from build123d import *

# Parameters (mm, degrees)
SKETCH1_R          = 2.54
EXTRUDE1_DEPTH     = 30.48
SKETCH2_W          = 2.032
SKETCH2_H          = 9.951877561
SKETCH2_W_2        = 1.949333431
SKETCH2_H_2        = 9.106721584
CUT_EXTRUDE1_DEPTH = 10.16
SKETCH4_R          = 1.524
CUT_EXTRUDE2_DEPTH = 10


with BuildPart() as part:
    # Sketch1 → Extrude1 (new body)
    with BuildSketch(Plane(origin=(0, 0, 0), x_dir=(1, 0, 0), z_dir=(0, 1, 0))):
        Circle(SKETCH1_R)
    extrude(amount=EXTRUDE1_DEPTH)

    # Sketch2 → Cut-Extrude1 (cut)
    with BuildSketch(Plane(origin=(0, 30.48, 0), x_dir=(-1, 0, 0), z_dir=(0, 1, 0))):
        with Locations((-2.54, 0.177802653)):
            Rectangle(SKETCH2_W, SKETCH2_H)
        with Locations((2.498666716, 0.600380641)):
            Rectangle(SKETCH2_W_2, SKETCH2_H_2)
    extrude(amount=-CUT_EXTRUDE1_DEPTH, mode=Mode.SUBTRACT)

    # Sketch4 → Cut-Extrude2 (cut)
    with BuildSketch(Plane.ZY.offset(1.524)):
        with Locations((0, 27.432)):
            Circle(SKETCH4_R)
    extrude(amount=-CUT_EXTRUDE2_DEPTH, mode=Mode.SUBTRACT)


solid = part.part
Work out the finished part from the listing and answer in its coordinate system (mm). A direction names the side the tool comes from. Round coordinates to 2 decimals unless told otherwise and drop trailing zeros. Write each loop counter-clockwise with the first axis right and the second up, starting at its lowest first coordinate (ties: lowest second). Pieces come first, ordered by that corner, then holes. Notation, with made-up numbers: (88, 75.25) -> (116, 75.25) arc R31 ccw to (116, 103.25) -> close; hole circle Ø1 at (-38, 2). An arc over 180 degrees is marked (long way). Answer as CSV lines item,"result". Start each with the question number.
(1) The part is cut by section B-B, the plane x = -0.05. Give the vertices of the cut face in (y, z), then the cut area to 3 significant figures.
(2) The part is cut by section A-A, the plane z = 0. Give the vertices of the cut face in (x, y).
(3) The part is cut by section C-C, the plane y = 25.5. Give the vertices of the cut face in (x, z).
(4) Find the intervals of material crossed by probe 1 along Y at (x, z) = (0.85, 0); probe 2 along Y at (x, z) = (-2.2, -1.15); probe 3 along Z at (x, y) = (-0.65, 26.5), in increasing order.
(5) The mould has two halves that part along Y. Classify faces 4 (the cylindrical face through (-0.021, 25.944, -0.33)), 5 (the flat face through (0, 30.48, 0)), 6 (the flat face through (-1.524, 25, 0)): +Y half, -Y half, draft (parallel to the pull), parting line (faces both ways), or undercut.
(6) Each of these flat-tipped pins is pushed along its axis until it touches: pin 1 (0.5 mm diameter, centred on x = -2, z = -0.5, fed in from +Y); pin 2 (1.5 mm diameter, centred on y = 9.5, z = -1.5, fed in from +X); pin 3 (1 mm diameter, centred on x = -2, y = 5.5, fed in from -Z). Where does it stop, or does it pass through?
(7) A tool of negligible diameter and unlimited length cuts with its end or side. For faces 1 (the flat face through (-2, 20.32, 0)), 2 (the cylindrical face through (2.423, 11.64, -0.763)), 3 (the flat face through (1.524, 25, 0)), from which of +Z, -Z, +X, -X, +Y, -Y can it reach the whole face along a straight path? Write none if from no direction.
(8) The part is cut by section D-D, the plane x = -1.15. Give the vertices of the cut face in (y, z).
Output values:
1,outline,"(0, -2.54) -> (30.48, -2.54) -> (30.48, 2.54) -> (0, 2.54) -> close; hole circle Ø3.05 at (27.43, 0)"
1,area,"148 mm²"
2,outline,"(-2.54, 0) -> (2.54, 0) -> (2.54, 20.32) -> (1.52, 20.32) -> (1.52, 25.91) -> (-1.52, 25.91) -> (-1.52, 20.32) -> (-2.54, 20.32) -> close; (-1.52, 28.96) -> (1.52, 28.96) -> (1.52, 30.48) -> (-1.52, 30.48) -> close"
3,outline,"(-1.52, -2.03) arc R2.54 ccw to (1.52, -2.03) -> (1.52, 2.03) arc R2.54 ccw to (-1.52, 2.03) -> close"
4,probe 1,"y = 0 to 25.91, 28.96 to 30.48"
4,probe 2,"y = 0 to 20.32"
4,probe 3,"z = -2.46 to -1.21, 1.21 to 2.46"
5,face 4,"undercut"
5,face 5,"+Y half"
5,face 6,"draft"
6,pin 1,"stops at y = 20.32"
6,pin 2,"stops at x = 2.43"
6,pin 3,"stops at z = -2.05"
7,face 1,"+Z, -Z, -X, +Y"
7,face 2,"+Y, -Y"
7,face 3,"+Z, -Z, +X, +Y"
8,outline,"(0, -2.26) -> (30.48, -2.26) -> (30.48, 2.26) -> (0, 2.26) -> close; hole circle Ø3.05 at (27.43, 0)"
